Check sheet for the drawn part. Datum: minimum x, y, z corner. Units: mm. A direction names the side the tool comes from. Give positions to 0.01 mm unless a question says otherwise; leave off trailing zeros. Write each loop counter-clockwise with the first axis right and the second up, starting at its lowest first coordinate (ties: lowest second). Pieces come first, ordered by that corner, then holes. Notation, with made-up numbers: (18.5, 23) -> (50.5, 23) arc R20 ccw to (50.5, 35) -> close; hole circle Ø4 at (-2.75, 2.5). An arc over 180 degrees is marked (long way). Write item = value, one per line. Start each with the question number.
1. Thickness scan on line 1 along Y through (x, z) = (1.75, 3.5); line 2 along X through (y, z) = (2, 2.5) (1 decimal); line 3 along X through (y, z) = (7, 1.5). Record the ranges inside material, lowest first.
2. Set-up check for the marked faces 1, 2 and 3: record each of +Z, -Z, +X, -X, +Y, -Y from which the full face is reachable in a straight line by a thin tool's end or side.
3. Cross-section at D-D, the plane y = 3. Record the cut outline in (x, z).
4. Cross-section at C-C, the plane z = 3.5. Record the cut outline in (x, y), plus the area to 3 significant figures.
5. Cross-section at B-B, the plane x = 3.25. Record the cut outline in (y, z).
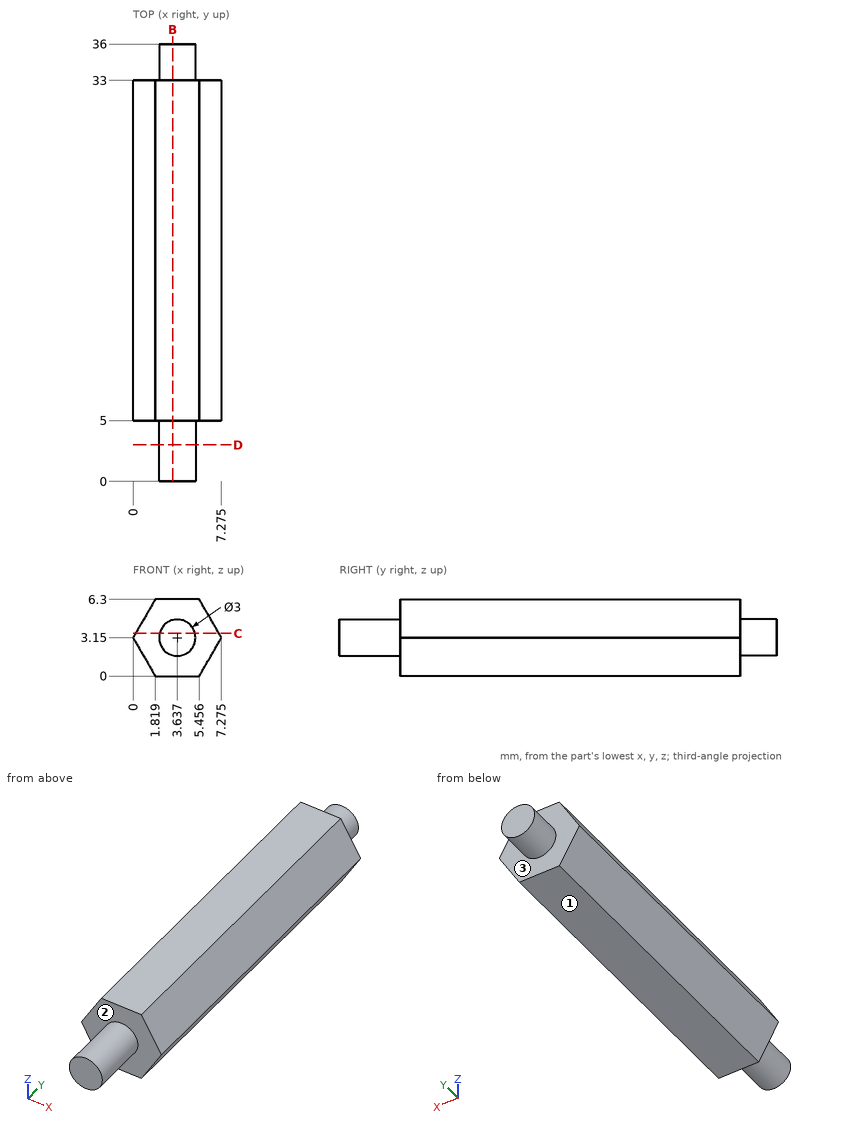
Answers:
q1.line_1 = 5 to 33
q1.line_2 = 2.3 to 5
q1.line_3 = 0.95 to 6.32
q2.face_1 = -Z, +X, -X, +Y, -Y
q2.face_2 = -Y
q2.face_3 = +Y
q3.outline = circle Ø3 at (3.64, 3.15)
q4.outline = (0.2, 5) -> (2.18, 5) -> (2.18, 0) -> (5.1, 0) -> (5.1, 5) -> (7.07, 5) -> (7.07, 33) -> (5.1, 33) -> (5.1, 36) -> (2.18, 36) -> (2.18, 33) -> (0.2, 33) -> close
q4.area = 216 mm^2
q5.outline = (0, 1.7) -> (5, 1.7) -> (5, 0) -> (33, 0) -> (33, 1.7) -> (36, 1.7) -> (36, 4.6) -> (33, 4.6) -> (33, 6.3) -> (5, 6.3) -> (5, 4.6) -> (0, 4.6) -> close
